```python
from build123d import *

# Parameters (mm, degrees)
CROQUIS3_W              = 160
CROQUIS3_H              = 22
SALIENTE_EXTRUIR1_DEPTH = 89
CROQUIS6_W              = 50
CROQUIS6_H              = 8
CORTAR_EXTRUIR1_DEPTH   = 69
REDONDEO1_R             = 20
REDONDEO2_R             = 20
CROQUIS7_R              = 17.5
SALIENTE_EXTRUIR3_DEPTH = 15
CROQUIS8_R              = 32
CROQUIS8_R_2            = 17.5
SALIENTE_EXTRUIR4_DEPTH = 49
CROQUIS9_W              = 45
CROQUIS9_H              = 25
CROQUIS9_W_2            = 16
SALIENTE_EXTRUIR5_DEPTH = 42
REDONDEO3_R             = 8
REDONDEO4_R             = 8
CROQUIS10_W             = 45
CROQUIS10_H             = 10


with BuildPart() as part:
    # Croquis3 → Saliente-Extruir1 (new body)
    with BuildSketch(Plane.XY):
        with Locations((80, 11)):
            Rectangle(CROQUIS3_W, CROQUIS3_H)
    extrude(amount=-SALIENTE_EXTRUIR1_DEPTH)

    # Croquis6 → Cortar-Extruir1 (cut)
    with BuildSketch(Plane.XY):
        with Locations((80, 18)):
            Rectangle(CROQUIS6_W, CROQUIS6_H)
    extrude(amount=-CORTAR_EXTRUIR1_DEPTH, mode=Mode.SUBTRACT)

    # Redondeo1
    redondeo1_edges = [part.edges().sort_by_distance(p)[0] for p in [
        (160, 11, 0),
    ]]
    fillet(redondeo1_edges, radius=REDONDEO1_R)

    # Redondeo2
    redondeo2_edges = [part.edges().sort_by_distance(p)[0] for p in [
        (0, 11, 0),
    ]]
    fillet(redondeo2_edges, radius=REDONDEO2_R)



with BuildPart() as body_2:
    # Croquis7 → Saliente-Extruir3 (new body)
    with BuildSketch(Plane(origin=(0, 0, -89), x_dir=(-1, 0, 0), z_dir=(0, 0, -1))):
        with BuildLine():
            Line((0, 22), (-160, 22))
            Line((-160, 22), (-160, 75))
            ThreePointArc((-160, 75), (-143.127064471, 103.198792891), (-110.301754969, 101.660309879))
            Line((-110.301754969, 101.660309879), (-5.363158113, 31.997616205))
            ThreePointArc((-5.363158113, 31.997616205), (-1.425452666, 27.672649177), (0, 22))
        make_face()
        with Locations((-128, 75)):
            Circle(CROQUIS7_R, mode=Mode.SUBTRACT)
    extrude(amount=-SALIENTE_EXTRUIR3_DEPTH)

    # Croquis8 → Saliente-Extruir4 (add)
    with BuildSketch(Plane.XY.offset(-74)):
        with Locations((128, 75)):
            Circle(CROQUIS8_R)
        with Locations(Location((128, 75, 0), (0, 0, 180))):
            Circle(CROQUIS8_R_2, mode=Mode.SUBTRACT)
    extrude(amount=SALIENTE_EXTRUIR4_DEPTH)


with BuildPart() as part_1:
    add(part.part)

    add(body_2.part)  # Saliente-Extruir5 merges body 2
    # Croquis9 → Saliente-Extruir5 (add)
    with BuildSketch(Plane.XY.offset(-74)):
        with Locations((22.5, 34.5)):
            Rectangle(CROQUIS9_W, CROQUIS9_H)
        with Locations((128, 34.5)):
            Rectangle(CROQUIS9_W_2, CROQUIS9_H)
    extrude(amount=SALIENTE_EXTRUIR5_DEPTH)

    # Redondeo3
    redondeo3_edges = [part_1.edges().sort_by_distance(p)[0] for p in [
        (136, 33.008066615, -32),
    ]]
    fillet(redondeo3_edges, radius=REDONDEO3_R)

    # Redondeo4
    redondeo4_edges = [part_1.edges().sort_by_distance(p)[0] for p in [
        (120, 33.008066615, -32),
    ]]
    fillet(redondeo4_edges, radius=REDONDEO4_R - 0.0001)  # a hair under: the kernel refuses the full size

    # Croquis10 → Cortar-Revolución1 (revolve, cut)
    with BuildSketch(Plane.XY.offset(-53)):
        with Locations((22.5, 42)):
            Rectangle(CROQUIS10_W, CROQUIS10_H)
    revolve(axis=Axis((45, 47, -53), (-1, 0, 0)), mode=Mode.SUBTRACT)

    # Croquis14 → Cortar-Revolución2 (revolve, cut)
    with BuildSketch(Plane.XY.offset(-53), mode=Mode.PRIVATE) as cortar_revoluci_n2_sk:
        Polygon((70, 14), (70, 6), (75, 6), (75, -24.123756484), (80, -24.123756484), (80, 14), align=None)
    revolve(cortar_revoluci_n2_sk.sketch.rotate(Axis((80, 14, -53), (0, -1, 0)), 270), axis=Axis((80, 14, -53), (0, -1, 0)), mode=Mode.SUBTRACT)

    # Croquis16 → Cortar-Revolución3 (revolve, cut)
    with BuildSketch(Plane.XY.offset(-20)):
        Polygon((10, 22), (10, 14), (15, 14), (15, -14.561047929), (20, -14.561047929), (20, 22), align=None)
    revolve(axis=Axis((20, 59.332394472, -20), (0, -1, 0)), mode=Mode.SUBTRACT)

    # Croquis17 → Cortar-Revolución4 (revolve, cut)
    with BuildSketch(Plane.XY.offset(-20), mode=Mode.PRIVATE) as cortar_revoluci_n4_sk:
        Polygon((140, 22), (150, 22), (150, 14), (145, 14), (145, 0), (140, 0), align=None)
    revolve(cortar_revoluci_n4_sk.sketch.rotate(Axis((140, -22.856797355, -20), (0, 1, 0)), 90), axis=Axis((140, -22.856797355, -20), (0, 1, 0)), mode=Mode.SUBTRACT)


solid = part_1.part
```
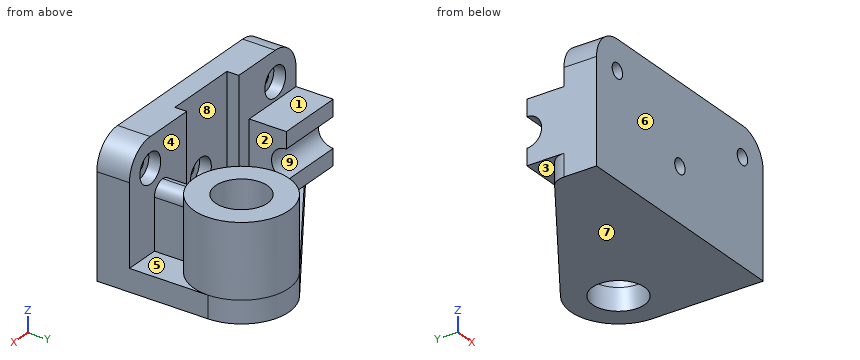
Source: CAD feature listing. Evaluate the final solid. Frame: model axes, mm. Face numbers are marked on the shaded views. A direction names the side the tool comes from. Coordinates: 2 decimals unless noted, no trailing zeros. Loops run counter-clockwise (first coordinate to the right, second up) from the corner with the lowest first, then second, coordinate; pieces in that order, holes last. Notation, with made-up numbers: M -36,58.25 L -14,58.25 A20 ccw -14,92.25 Z; hole C 78,-26 d6. An arc over 180 degrees is marked long. Use CSV: the item, a comma, the result in double quotes.
(1) Reachability of the marked faces 1, 2, 3, 4 and 5 from +Z, -Z, +X, -X, +Y, -Y: full face, straight path, thin tool, end or side. Return the list, or none.
Answers follow:
face 1,"+Z, -X, +Y"
face 2,"+Z, +Y"
face 3,"-Z, -X, +Y"
face 4,"+Z"
face 5,"+Z, +X"
(2) Contact query for flat-ended pins moving along their axis: pin 1 (10 mm diameter, centred on x = 24.5, z = -60, fed in from +Y); pin 2 (8 mm diameter, centred on x = 71.5, z = -62.5, fed in from -Y); pin 3 (19 mm diameter, centred on x = 154, y = 44, fed in from +Z); pin 4 (6 mm diameter, centred on x = 140.5, z = -44, fed in from +Y). Output: stop coordinate, or through.
Answers follow:
pin 1,"y = 47"
pin 2,"y = 0"
pin 3,"z = -25"
pin 4,"y = 105.56"
(3) Cut plane C-C on x = 80. Return loops of the section in (y, z).
Answers follow:
outline,"M 0,-89 L 81.54,-89 L 81.54,-74 L 22,-74 L 22,-69 L 14,-69 L 14,-63 L 6,-63 L 6,-58 L 0,-58 Z; M 0,-48 L 6,-48 L 6,-43 L 14,-43 L 14,0 L 0,0 Z"
(4) Draft query along Y for the marked faces 6, 7, 8 and 9. Return one class per face: pulls with the +Y half, pulls with the -Y half, needs draft (parallel to the pull), parting line crosses it, or undercut.
Answers follow:
face 6,"pulls with the -Y half"
face 7,"needs draft"
face 8,"undercut"
face 9,"pulls with the +Y half"
(5) Cut plane B-B on z = -22.5. Return loops of the section in (x, y).
Answers follow:
outline,"M 0,0 L 15.67,0 L 15.67,14 L 10.32,14 L 10.32,22 L 0,22 Z; M 24.33,0 L 135.67,0 L 135.67,14 L 130.32,14 L 130.32,22 L 105,22 L 105,14 L 55,14 L 55,22 L 29.68,22 L 29.68,14 L 24.33,14 Z; M 144.33,0 L 160,0 L 160,22 L 149.68,22 L 149.68,14 L 144.33,14 Z"
(6) Line query: line 1 (X direction, y = 23.5, z = -71); line 2 (Z direction, x = 20, y = 10); line 3 (X direction, y = 8.25, z = -53). Output: solid intervals per line, ascending. Write a range as [from, to].
Answers follow:
line 1,"[0, 45], [120, 136]"
line 2,"[-89, -25], [-15, 0]"
line 3,"[0, 70], [90, 160]"
(7) Cut plane A-A on z = -54. Return loops of the section in (x, y).
Answers follow:
outline,"M 0,0 L 75.1,0 L 75.1,6 L 70.05,6 L 70.05,14 L 55,14 L 55,22 L 45,22 L 45,37.05 L 0,37.05 Z; M 84.9,0 L 160,0 L 160,22 L 136,22 L 136,44.02 A32 ccw long 120,44.02 L 120,22 L 105,22 L 105,14 L 89.95,14 L 89.95,6 L 84.9,6 Z; hole C 128,75 d35"
(8) Cut plane D-D on y = 94.5. Return loops of the section in (x, z).
Answers follow:
outline,"M 99.52,-89 L 153.37,-89 L 153.37,-25 L 102.63,-25 L 102.63,-74 L 99.52,-74 Z"
